Geometry check sheet. Reference: the model listing, model coordinates, mm. Give positions to 0.01 mm unless a question says otherwise; leave off trailing zeros. Write each loop counter-clockwise with the first axis right and the second up, starting at its lowest first coordinate (ties: lowest second). Pieces come first, ordered by that corner, then holes.
(1) Cross-section at D-D (x = 11). Record the boundary of the cut face in (y, z).
(2) Cross-section at B-B (y = 3.75). Record the boundary of the cut face in (x, z).
(3) Thickness scan on line 1 along X through (y, z) = (6.25, -45); line 2 along X through (y, z) = (3.5, -45); line 3 along Z through (x, y) = (11, 3.5). Record the ranges inside material, lowest first.
(4) Cross-section at A-A (z = -5). Record the boundary of the cut face in (x, y), and give its area (3 significant figures).
(5) Mould release check, pull along Z, two halves, no side actions. Record for faces 1 (the flat face through (0.21, 6.344, -49.014)), 2 (the flat face through (-14.014, 6.344, -24.65)), 3 (the cylindrical face through (-10.04, 3.95, -46.65)), 4 (the cylindrical face through (-10.04, 3.95, -6.65)): +Z half, -Z half, draft (parallel to the pull), parting line (faces both ways), or undercut.
(6) Cross-section at C-C (z = -30.5). Record the boundary of the cut face in (x, y).
```python
from build123d import *
from OCP.BRepAlgoAPI import BRepAlgoAPI_Cut
from OCP.TopTools import TopTools_ListOfShape

# Parameters (mm, degrees)
BOSS_EXTRUDE1_DEPTH = 50
SKETCH4_R           = 1.65
CUT_EXTRUDE1_DEPTH  = 7.792432
CHAMFER1_SIZE       = 2
CHAMFER1_SIZE2      = 2.856296013


with BuildPart() as part:
    # Sketch2 → Boss-Extrude1 (new body)
    with BuildSketch(Plane.XY):
        with BuildLine():
            Line((5.230022165, 0), (15, 0))
            Line((15, 0), (15, 7.792432351))
            Line((15, 7.792432351), (-15, 7.792432351))
            Line((-15, 7.792432351), (-15, 0))
            Line((-15, 0), (-5.230022165, 0))
            ThreePointArc((-5.230022165, 0), (0, 4.792432351), (5.230022165, 0))
        make_face()
    extrude(amount=-BOSS_EXTRUDE1_DEPTH)


with BuildPart() as cut_extrude1_tool:
    # Sketch4 → Cut-Extrude1 (new body)
    with BuildSketch(Plane(origin=(0, 7.792432351, 0), x_dir=(1, 0, 0), z_dir=(0, 1, 0))):
        with Locations(Location((-10.115011082, 45, 0), (0, 0, 270))):
            Circle(SKETCH4_R)
        with Locations(Location((-10.115011082, 5, 0), (0, 0, 270))):
            Circle(SKETCH4_R)
        with Locations(Location((10.115011082, 45, 0), (0, 0, 270))):
            Circle(SKETCH4_R)
        with Locations(Location((10.115011082, 5, 0), (0, 0, 270))):
            Circle(SKETCH4_R)
    extrude(amount=-CUT_EXTRUDE1_DEPTH)


with BuildPart() as part_1:
    add(part.part)

    # Cut-Extrude1: cut by cut_extrude1_tool, with a tolerance
    cut_extrude1_stock = TopTools_ListOfShape()
    cut_extrude1_stock.Append(part_1.part.wrapped)
    cut_extrude1_tools = TopTools_ListOfShape()
    cut_extrude1_tools.Append(cut_extrude1_tool.part.wrapped)
    cut_extrude1_cut = BRepAlgoAPI_Cut()
    cut_extrude1_cut.SetArguments(cut_extrude1_stock)
    cut_extrude1_cut.SetTools(cut_extrude1_tools)
    cut_extrude1_cut.SetFuzzyValue(0.00001)
    cut_extrude1_cut.Build()
    add(Compound.cast(cut_extrude1_cut.Shape()).solids(), mode=Mode.REPLACE)

    # Chamfer1
    chamfer1_edges = [part_1.edges().sort_by_distance(p)[0] for p in [
        (0, 7.792432351, 0),
        (15, 7.792432351, -25),
        (0, 7.792432351, -50),
        (-15, 7.792432351, -25),
    ]]
    chamfer1_side = [part_1.faces().sort_by_distance(p)[0] for p in [
        (0, 7.792432351, -25),
    ]]
    chamfer(chamfer1_edges, length=CHAMFER1_SIZE, length2=CHAMFER1_SIZE2, reference=chamfer1_side[0])


solid = part_1.part
```
Reply:
1. outline: (0, -50) - (4.94, -50) - (7.79, -48) - (7.79, -46.39) - (0, -46.39) - close; (0, -43.61) - (7.79, -43.61) - (7.79, -6.39) - (0, -6.39) - close; (0, -3.61) - (7.79, -3.61) - (7.79, -2) - (4.94, 0) - (0, 0) - close
2. outline: (-15, -50) - (-3.14, -50) - (-3.14, 0) - (-15, 0) - close; (3.14, -50) - (15, -50) - (15, 0) - (3.14, 0) - close; hole circle Ø3.3 at (-10.12, -45); hole circle Ø3.3 at (-10.12, -5); hole circle Ø3.3 at (10.12, -45); hole circle Ø3.3 at (10.12, -5)
3. line 1: x = -14.08 to -11.77, -8.47 to 8.47, 11.77 to 14.08
3. line 2: x = -15 to -11.77, -8.47 to -3.45, 3.45 to 8.47, 11.77 to 15
3. line 3: z = -50 to -46.39, -43.61 to -6.39, -3.61 to 0
4. outline: (-15, 0) - (-11.77, 0) - (-11.77, 7.79) - (-13, 7.79) - (-15, 4.94) - close; (-8.47, 0) - (-5.23, 0) arc R5.25 cw to (5.23, 0) - (8.47, 0) - (8.47, 7.79) - (-8.47, 7.79) - close; (11.77, 0) - (15, 0) - (15, 4.94) - (13, 7.79) - (11.77, 7.79) - close
4. area: 138 mm2
5. face 1: -Z half
5. face 2: draft
5. face 3: undercut
5. face 4: undercut
6. outline: (-15, 0) - (-5.23, 0) arc R5.25 cw to (5.23, 0) - (15, 0) - (15, 4.94) - (13, 7.79) - (-13, 7.79) - (-15, 4.94) - close
